Read the model definition and answer for the solid it produces. Units are mm, in the model's axes. Round coordinates to 2 decimals unless told otherwise and drop trailing zeros. Loops run counter-clockwise (first coordinate to the right, second up) from the corner with the lowest first, then second, coordinate; pieces in that order, holes last. Notation, with made-up numbers: (45.25, 1.25) -> (95.25, 1.25) arc R20 ccw to (95.25, 14.25) -> close; hole circle Ø5 at (59, 46.5). An arc over 180 degrees is marked (long way). Put each result on its own line as item: value.
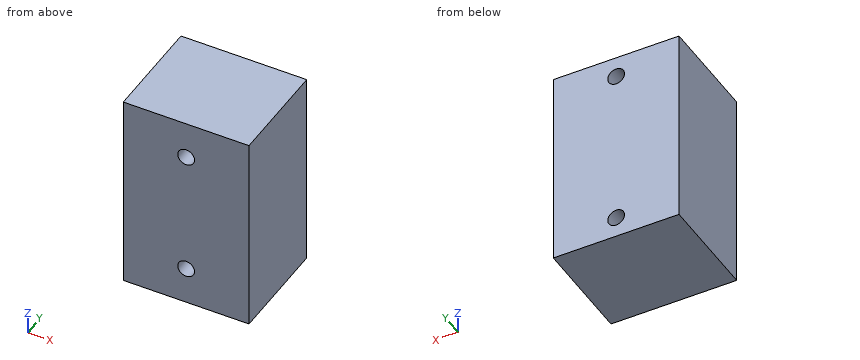
from build123d import *

# Parameters (mm, degrees)
SKETCH1_W           = 30
SKETCH1_H           = 25
BOSS_EXTRUDE1_DEPTH = 48
SKETCH2_R           = 2
CUT_EXTRUDE3_DEPTH  = 10
SKETCH3_R           = 2
CUT_EXTRUDE4_DEPTH  = 10


with BuildPart() as part:
    # Sketch1 → Boss-Extrude1 (new body)
    with BuildSketch(Plane.XY):
        with Locations((15, 12.5)):
            Rectangle(SKETCH1_W, SKETCH1_H)
    extrude(amount=BOSS_EXTRUDE1_DEPTH)

    # Sketch2 → Cut-Extrude3 (cut)
    with BuildSketch(Plane(origin=(0, 25, 0), x_dir=(1, 0, 0), z_dir=(0, 1, 0))):
        with Locations(Location((15, -5, 0), (0, 0, 180))):
            Circle(SKETCH2_R)
        with Locations(Location((15, -43, 0), (0, 0, 180))):
            Circle(SKETCH2_R)
    extrude(amount=-CUT_EXTRUDE3_DEPTH, mode=Mode.SUBTRACT)

    # Sketch3 → Cut-Extrude4 (cut)
    with BuildSketch(Plane.XZ):
        with Locations(Location((15, 39, 0), (0, 0, 270))):
            Circle(SKETCH3_R)
        with Locations(Location((15, 9, 0), (0, 0, 270))):
            Circle(SKETCH3_R)
    extrude(amount=-CUT_EXTRUDE4_DEPTH, mode=Mode.SUBTRACT)


solid = part.part
Item 1: The part is cut by section C-C (x = 15). Determine the outline of the cut face in (y, z), then the cut area to 3 significant figures.
Derived:
outline: (0, 0) -> (25, 0) -> (25, 3) -> (15, 3) -> (15, 7) -> (25, 7) -> (25, 41) -> (15, 41) -> (15, 45) -> (25, 45) -> (25, 48) -> (0, 48) -> (0, 41) -> (10, 41) -> (10, 37) -> (0, 37) -> (0, 11) -> (10, 11) -> (10, 7) -> (0, 7) -> close
area: 1,040 mm^2
Item 2: The part is cut by section A-A (z = 9). Determine the outline of the cut face in (x, y).
Derived:
outline: (0, 0) -> (13, 0) -> (13, 10) -> (17, 10) -> (17, 0) -> (30, 0) -> (30, 25) -> (0, 25) -> close
Item 3: The part is cut by section B-B (y = 17). Determine the outline of the cut face in (x, z), then the cut area to 3 significant figures.
Derived:
outline: (0, 0) -> (30, 0) -> (30, 48) -> (0, 48) -> close; hole circle Ø4 at (15, 5); hole circle Ø4 at (15, 43)
area: 1,410 mm^2
Item 4: Find the intervals of material crossed by line 1 along Z through (x, y) = (15, 22.75); line 2 along Z through (x, y) = (14, 5.5); line 3 along Y through (x, z) = (13.25, 43), in increasing order.
Derived:
line 1: z = 0 to 3, 7 to 41, 45 to 48
line 2: z = 0 to 7.27, 10.73 to 37.27, 40.73 to 48
line 3: y = 0 to 15
Item 5: A flat-ended cylindrical pin translates along its axis: pin 1 Ø2.5 at (x, z) = (15, 39) entering from -Y. Find the tip coordinate at first contact, or state that the pin passes through.
Derived:
pin 1: stops at y = 10
